Source: three-view drawing plus pictorial views. Frame: mm from the lowest corner of the part. A direction names the side the tool comes from. Coordinates: 2 decimals unless noted, no trailing zeros. Write each loop counter-clockwise with the first axis right and the second up, starting at its lowest first coordinate (ties: lowest second). Pieces come first, ordered by that corner, then holes.
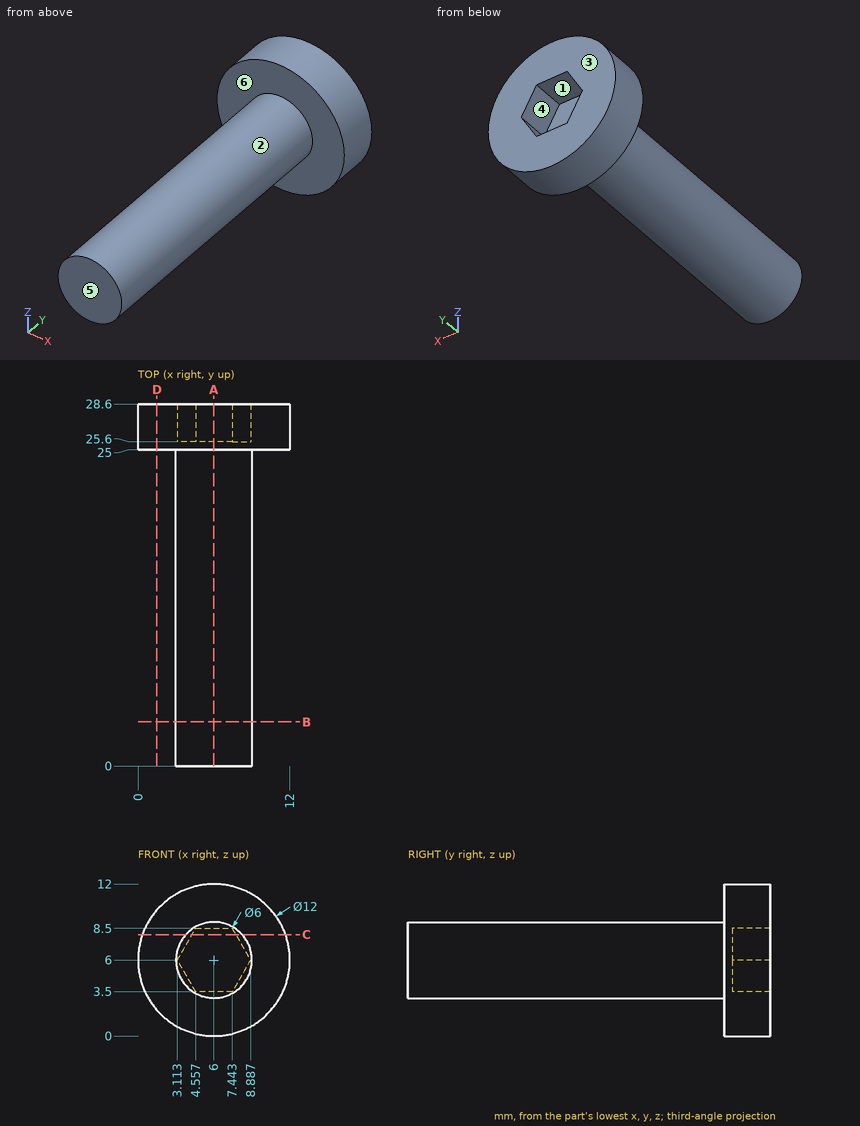
Item 1: Section query C-C, the plane z = 8. Return loops of the section in (x, y), then the cut area to 3 significant figures.
Item 2: Section query D-D, the plane x = 1.5. Return loops of the section in (y, z), then the cut area to 3 significant figures.
Item 3: Section query B-B, the plane y = 3.5. Return loops of the section in (x, z).
Item 4: Access query for the marked faces 4, 5 and 6. Directions: +Z, -Z, +X, -X, +Y, -Y. A direction counts if a zero-diameter tool reaches every point of the face in a straight line with its end or side. Return the directions, or none.
Item 5: Pin query (flat end, axial travel): pin 1 Ø2.5 at (x, z) = (6.5, 6.5) entering from +Y; pin 2 Ø6 at (y, z) = (15.5, 5) entering from -X; pin 3 Ø6 at (x, y) = (8.5, 10.5) entering from -Z. Return the tip coordinate at first contact, or that it passes through.
Item 6: Material intervals for line 1 (Y direction, x = 11.5, z = 7.25); line 2 (Y direction, x = 6.25, z = 3.75); line 3 (Z direction, x = 6, y = 6.75), sorted ascending.
Item 7: Pull-direction query (Z, two-part tool) for the marked faces 1, 2 and 3; classes: released by +Z, released by -Z, zero draft, split by the parting line, or undercut.
Item 8: Section query A-A, the plane x = 6. Return loops of the section in (y, z).
The answers:
1. outline: (0.34, 25) - (3.76, 25) - (3.76, 0) - (8.24, 0) - (8.24, 25) - (11.66, 25) - (11.66, 28.6) - (7.73, 28.6) - (7.73, 25.6) - (4.27, 25.6) - (4.27, 28.6) - (0.34, 28.6) - close
1. area: 142 mm2
2. outline: (25, 2.03) - (28.6, 2.03) - (28.6, 9.97) - (25, 9.97) - close
2. area: 28.6 mm2
3. outline: circle Ø6 at (6, 6)
4. face 4: +Y
4. face 5: +Z, -Z, +X, -X, -Y
4. face 6: -Y
5. pin 1: stops at y = 25.6
5. pin 2: stops at x = 3
5. pin 3: stops at z = 3
6. line 1: y = 25 to 28.6
6. line 2: y = 0 to 25.6
6. line 3: z = 3 to 9
7. face 1: undercut
7. face 2: split by the parting line
7. face 3: zero draft
8. outline: (0, 3) - (25, 3) - (25, 0) - (28.6, 0) - (28.6, 3.5) - (25.6, 3.5) - (25.6, 8.5) - (28.6, 8.5) - (28.6, 12) - (25, 12) - (25, 9) - (0, 9) - close
